Build history of the part. All positions in model axes, mm. Face numbers are marked on the shaded views. A direction names the side the tool comes from. Coordinates: 2 decimals unless noted, no trailing zeros. Order: outer loops, then holes, each group sorted by start corner. A loop starts at its lowest first (then second) coordinate and runs counter-clockwise, first axis right, second up. Notation, with made-up numbers: (12, 16.25) - (65, 16.25) arc R30 ccw to (65, 41.25) - close; hole circle Ø9 at (-29.5, 57). An arc over 180 degrees is marked (long way). One line per item, written item: value.
from build123d import *

# Parameters (mm, degrees)
SKETCH_1_R          = 1.2
EXTRUDE_1_DEPTH     = 27.5
CUT_EXTRUDE_1_DEPTH = 28.5


with BuildPart() as part:
    # 草图1 → 凸台-拉伸1 (new body)
    with BuildSketch(Plane.XY):
        with BuildLine():
            Line((15.356969673, 30.298929166), (13.674015522, 31.101791788))
            ThreePointArc((13.674015522, 31.101791788), (11.571454033, 31.125101256), (10.194791162, 29.535727958))
            ThreePointArc((10.194791162, 29.535727958), (6.381394442, 23.991783581), (0, 21.857511157))
            ThreePointArc((0, 21.857511157), (-6.773355282, 24.696305694), (-9.498676044, 31.516109427))
            ThreePointArc((-9.498676044, 31.516109427), (-9.831389744, 32.178886119), (-10.565560882, 32.28359567))
            Line((-10.565560882, 32.28359567), (-12.323298779, 31.661276982))
            ThreePointArc((-12.323298779, 31.661276982), (-13.826516548, 30.191023779), (-13.676107562, 28.09371949))
            ThreePointArc((-13.676107562, 28.09371949), (-12.45242558, 21.477080146), (-15.455594359, 15.455594359))
            ThreePointArc((-15.455594359, 15.455594359), (-22.252410678, 12.673439775), (-29.001832935, 15.568676449))
            ThreePointArc((-29.001832935, 15.568676449), (-29.705750942, 15.802066229), (-30.298929166, 15.356969673))
            Line((-30.298929166, 15.356969673), (-31.101791788, 13.674015522))
            ThreePointArc((-31.101791788, 13.674015522), (-31.125101256, 11.571454033), (-29.535727958, 10.194791162))
            ThreePointArc((-29.535727958, 10.194791162), (-23.991783581, 6.381394442), (-21.857511157, 0))
            ThreePointArc((-21.857511157, 0), (-24.696305694, -6.773355282), (-31.516109427, -9.498676044))
            ThreePointArc((-31.516109427, -9.498676044), (-32.178886119, -9.831389744), (-32.28359567, -10.565560882))
            Line((-32.28359567, -10.565560882), (-31.661276982, -12.323298779))
            ThreePointArc((-31.661276982, -12.323298779), (-30.191023779, -13.826516548), (-28.09371949, -13.676107562))
            ThreePointArc((-28.09371949, -13.676107562), (-21.477080146, -12.45242558), (-15.455594359, -15.455594359))
            ThreePointArc((-15.455594359, -15.455594359), (-12.673439775, -22.252410678), (-15.568676449, -29.001832935))
            ThreePointArc((-15.568676449, -29.001832935), (-15.802066229, -29.705750942), (-15.356969673, -30.298929166))
            Line((-15.356969673, -30.298929166), (-13.674015522, -31.101791788))
            ThreePointArc((-13.674015522, -31.101791788), (-11.571454033, -31.125101256), (-10.194791162, -29.535727958))
            ThreePointArc((-10.194791162, -29.535727958), (-6.381394442, -23.991783581), (0, -21.857511157))
            ThreePointArc((0, -21.857511157), (6.773355282, -24.696305694), (9.498676044, -31.516109427))
            ThreePointArc((9.498676044, -31.516109427), (9.831389744, -32.178886119), (10.565560882, -32.28359567))
            Line((10.565560882, -32.28359567), (12.323298779, -31.661276982))
            ThreePointArc((12.323298779, -31.661276982), (13.826516548, -30.191023779), (13.676107562, -28.09371949))
            ThreePointArc((13.676107562, -28.09371949), (12.45242558, -21.477080146), (15.455594359, -15.455594359))
            ThreePointArc((15.455594359, -15.455594359), (22.252410678, -12.673439775), (29.001832935, -15.568676449))
            ThreePointArc((29.001832935, -15.568676449), (29.705750942, -15.802066229), (30.298929166, -15.356969673))
            Line((30.298929166, -15.356969673), (31.101791788, -13.674015522))
            ThreePointArc((31.101791788, -13.674015522), (31.125101256, -11.571454033), (29.535727958, -10.194791162))
            ThreePointArc((29.535727958, -10.194791162), (23.991783581, -6.381394442), (21.857511157, 0))
            ThreePointArc((21.857511157, 0), (24.696305694, 6.773355282), (31.516109427, 9.498676044))
            ThreePointArc((31.516109427, 9.498676044), (32.178886119, 9.831389744), (32.28359567, 10.565560882))
            Line((32.28359567, 10.565560882), (31.661276982, 12.323298779))
            ThreePointArc((31.661276982, 12.323298779), (30.191023779, 13.826516548), (28.09371949, 13.676107562))
            ThreePointArc((28.09371949, 13.676107562), (21.477080146, 12.45242558), (15.455594359, 15.455594359))
            ThreePointArc((15.455594359, 15.455594359), (12.673439775, 22.252410678), (15.568676449, 29.001832935))
            ThreePointArc((15.568676449, 29.001832935), (15.802066229, 29.705750942), (15.356969673, 30.298929166))
        make_face()
        with Locations((12.597590691, 28.845398741)):
            Circle(SKETCH_1_R, mode=Mode.SUBTRACT)
        with Locations((29.304618859, 11.488935252)):
            Circle(SKETCH_1_R, mode=Mode.SUBTRACT)
        with Locations((28.845398741, -12.597590691)):
            Circle(SKETCH_1_R, mode=Mode.SUBTRACT)
        with Locations((11.488935252, -29.304618859)):
            Circle(SKETCH_1_R, mode=Mode.SUBTRACT)
        with Locations((-12.597590691, -28.845398741)):
            Circle(SKETCH_1_R, mode=Mode.SUBTRACT)
        with Locations((-29.304618859, -11.488935252)):
            Circle(SKETCH_1_R, mode=Mode.SUBTRACT)
        with Locations((-28.845398741, 12.597590691)):
            Circle(SKETCH_1_R, mode=Mode.SUBTRACT)
        with Locations((-11.488935252, 29.304618859)):
            Circle(SKETCH_1_R, mode=Mode.SUBTRACT)
    extrude(amount=EXTRUDE_1_DEPTH)

    # 草图2 → 切除-拉伸1 (cut, through all)
    with BuildSketch(Plane(origin=(0, 0, 0), x_dir=(-1, 0, 0), z_dir=(0, 0, -1))):
        with BuildLine():
            ThreePointArc((20.657511157, 0), (21.762964244, -4.736525047), (24.85090733, -8.494357341))
            ThreePointArc((24.85090733, -8.494357341), (25.340600313, -10.218879989), (23.827990301, -11.181059043))
            ThreePointArc((23.827990301, -11.181059043), (18.843757471, -11.888077559), (14.607066222, -14.607066222))
            ThreePointArc((14.607066222, -14.607066222), (12.039510615, -18.737968576), (11.565827414, -23.578662769))
            ThreePointArc((11.565827414, -23.578662769), (10.692670984, -25.144349657), (8.942730853, -24.755136194))
            ThreePointArc((8.942730853, -24.755136194), (4.918408433, -21.730688948), (0, -20.657511157))
            ThreePointArc((0, -20.657511157), (-4.736525047, -21.762964244), (-8.494357341, -24.85090733))
            ThreePointArc((-8.494357341, -24.85090733), (-10.218879989, -25.340600313), (-11.181059043, -23.827990301))
            ThreePointArc((-11.181059043, -23.827990301), (-11.888077559, -18.843757471), (-14.607066222, -14.607066222))
            ThreePointArc((-14.607066222, -14.607066222), (-18.737968576, -12.039510615), (-23.578662769, -11.565827414))
            ThreePointArc((-23.578662769, -11.565827414), (-25.144349657, -10.692670984), (-24.755136194, -8.942730853))
            ThreePointArc((-24.755136194, -8.942730853), (-21.730688948, -4.918408433), (-20.657511157, 0))
            ThreePointArc((-20.657511157, 0), (-21.762964244, 4.736525047), (-24.85090733, 8.494357341))
            ThreePointArc((-24.85090733, 8.494357341), (-25.340600313, 10.218879989), (-23.827990301, 11.181059043))
            ThreePointArc((-23.827990301, 11.181059043), (-18.843757471, 11.888077559), (-14.607066222, 14.607066222))
            ThreePointArc((-14.607066222, 14.607066222), (-12.039510615, 18.737968576), (-11.565827414, 23.578662769))
            ThreePointArc((-11.565827414, 23.578662769), (-10.692670984, 25.144349657), (-8.942730853, 24.755136194))
            ThreePointArc((-8.942730853, 24.755136194), (-4.918408433, 21.730688948), (0, 20.657511157))
            ThreePointArc((0, 20.657511157), (4.736525047, 21.762964244), (8.494357341, 24.85090733))
            ThreePointArc((8.494357341, 24.85090733), (10.218879989, 25.340600313), (11.181059043, 23.827990301))
            ThreePointArc((11.181059043, 23.827990301), (11.888077559, 18.843757471), (14.607066222, 14.607066222))
            ThreePointArc((14.607066222, 14.607066222), (18.737968576, 12.039510615), (23.578662769, 11.565827414))
            ThreePointArc((23.578662769, 11.565827414), (25.144349657, 10.692670984), (24.755136194, 8.942730853))
            ThreePointArc((24.755136194, 8.942730853), (21.730688948, 4.918408433), (20.657511157, 0))
        make_face()
    extrude(amount=-CUT_EXTRUDE_1_DEPTH, mode=Mode.SUBTRACT)


solid = part.part
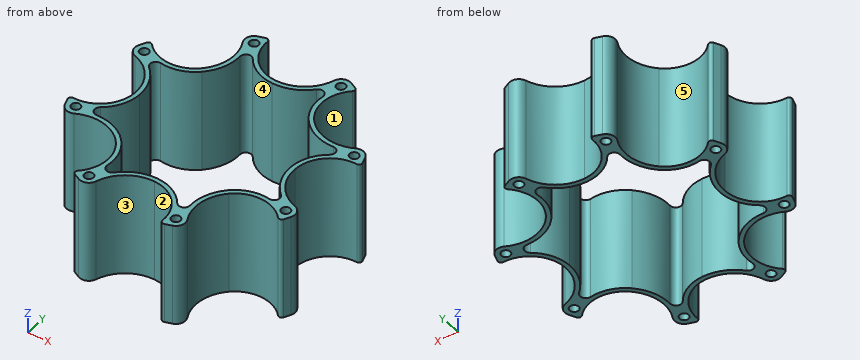
1. Probe line 1 along X through (y, z) = (-23, 17.5); line 2 along X through (y, z) = (0.5, 13.75); line 3 along Y through (x, z) = (15, 10.25). List the from-to ranges inside material, lowest first.
Values found:
line 1: x = -12.71 to -11.51, -7.06 to -4.79, 4.52 to 6.68, 11.15 to 12.35
line 2: x = -21.87 to -20.67, 20.67 to 21.87
line 3: y = -15.94 to -14.23, 14.23 to 15.94, 28.4 to 30.47
2. Two-plate mould, pull along X, no slides. Class the marked faces 1 and 2: pulls with the +X half, pulls with the -X half, needs draft (parallel to the pull), parting line crosses it, or undercut.
Values found:
face 1: pulls with the +X half
face 2: undercut
3. Band-saw the part on C-C, the plane z = 20. Count the separate pieces of the cut face and the enclosed holes in it, and give its area (3 significant figures).
Values found:
separate pieces: 1
enclosed holes: 9
area: 405 mm2
4. Band-saw the part on A-A, the plane y = 3. Give the cut face in (x, z) (3 decimals).
Values found:
outline: (-22.291, 0) - (-21.045, 0) - (-21.045, 27.5) - (-22.291, 27.5) - close; (21.087, 0) - (22.344, 0) - (22.344, 27.5) - (21.087, 27.5) - close
5. Flat gauge pins, fed straight in: P1, Ø10, axis at y = 22.5, z = 4.5, coming from the +X side; P2, Ø2, axis at y = -8.5, z = 15.5, coming from the +X side; P3, Ø4, axis at y = 23.5, z = 13, coming from the -X side. Where does each tip first touch, or does it go through?
Values found:
P1: stops at x = 14.31
P2: stops at x = 27.75
P3: stops at x = -12.66
6. 3-axis set-ups, long thin cutter, end or side, ignore diameter. For the marked faces 3, 4 and 5: which of +Z, -Z, +X, -X, +Y, -Y reach the whole face in a straight line?
Values found:
face 3: +Z, -Z, -Y
face 4: +Z, -Z
face 5: +Z, -Z, +Y
